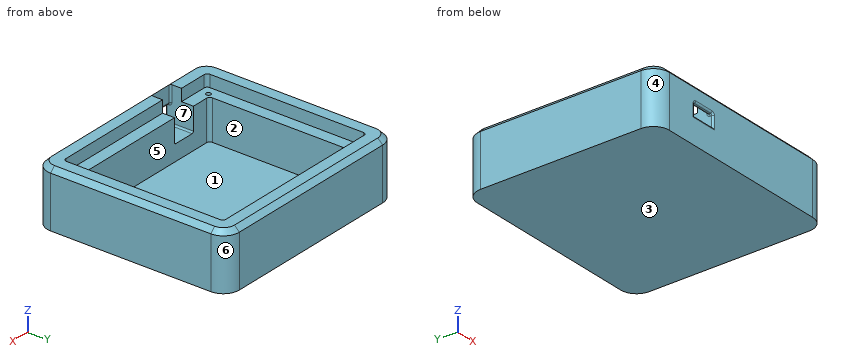
```python
from build123d import *

# Parameters (mm, degrees)
BASE_W              = 134
BASE_H              = 120.5
BASE_W_2            = 114
BASE_H_2            = 100.5
BASE_R              = 1.475
BASE_W_3            = 99
BASE_H_3            = 85.5
BOSS_EXTRUDE1_DEPTH = 3
BOSS_EXTRUDE2_START = 3
BASE_3_W            = 114
BASE_3_H            = 100.5
BASE_3_R            = 1.475
BASE_3_W_2          = 99
BASE_3_H_2          = 85.5
BOSS_EXTRUDE2_DEPTH = 25
BOSS_EXTRUDE3_START = 3
BASE_4_W            = 134
BASE_4_H            = 120.5
BASE_4_W_2          = 114
BASE_4_H_2          = 100.5
BOSS_EXTRUDE3_DEPTH = 32.5
SKETCH2_W           = 15
SKETCH2_H           = 14.5
CUT_EXTRUDE1_DEPTH  = 22.5
SKETCH3_W           = 15
SKETCH3_H           = 8
CUT_EXTRUDE2_DEPTH  = 3
FILLET1_R           = 10
FILLET2_R           = 2
FILLET3_R           = 1
CHAMFER1_SIZE       = 3


with BuildPart() as part:
    # Base → Boss-Extrude1 (new body)
    # profile 1 of 7: a face of its own
    with BuildSketch(Plane.XY):
        Rectangle(BASE_W, BASE_H)
        Rectangle(BASE_W_2, BASE_H_2, mode=Mode.SUBTRACT)
    # profile 2 of 7: a face of its own
    with BuildSketch(Plane.XY):
        Rectangle(BASE_W_2, BASE_H_2)
        with Locations((-51.5, -44.75)):
            Circle(BASE_R, mode=Mode.SUBTRACT)
        with Locations((51.5, -44.75)):
            Circle(BASE_R, mode=Mode.SUBTRACT)
        with Locations((51.5, 44.75)):
            Circle(BASE_R, mode=Mode.SUBTRACT)
        with Locations((-51.5, 44.75)):
            Circle(BASE_R, mode=Mode.SUBTRACT)
        Rectangle(BASE_W_3, BASE_H_3, mode=Mode.SUBTRACT)
    # profile 3 of 7: a face of its own
    with BuildSketch(Plane.XY):
        with Locations((51.5, -44.75)):
            Circle(BASE_R)
    # profile 4 of 7: a face of its own
    with BuildSketch(Plane.XY):
        with Locations((-51.5, 44.75)):
            Circle(BASE_R)
    # profile 5 of 7: a face of its own
    with BuildSketch(Plane.XY):
        with Locations((-51.5, -44.75)):
            Circle(BASE_R)
    # profile 6 of 7: a face of its own
    with BuildSketch(Plane.XY):
        with Locations((51.5, 44.75)):
            Circle(BASE_R)
    # profile 7 of 7: a face of its own
    with BuildSketch(Plane.XY):
        Rectangle(BASE_W_3, BASE_H_3)
    extrude(amount=BOSS_EXTRUDE1_DEPTH)

    # Base<3> → Boss-Extrude2 (add)
    with BuildSketch(Plane.XY.offset(BOSS_EXTRUDE2_START)):
        Rectangle(BASE_3_W, BASE_3_H)
        with Locations((-51.5, -44.75)):
            Circle(BASE_3_R, mode=Mode.SUBTRACT)
        with Locations((51.5, -44.75)):
            Circle(BASE_3_R, mode=Mode.SUBTRACT)
        with Locations((51.5, 44.75)):
            Circle(BASE_3_R, mode=Mode.SUBTRACT)
        with Locations((-51.5, 44.75)):
            Circle(BASE_3_R, mode=Mode.SUBTRACT)
        Rectangle(BASE_3_W_2, BASE_3_H_2, mode=Mode.SUBTRACT)
    extrude(amount=BOSS_EXTRUDE2_DEPTH)

    # Base<4> → Boss-Extrude3 (add)
    with BuildSketch(Plane.XY.offset(BOSS_EXTRUDE3_START)):
        Rectangle(BASE_4_W, BASE_4_H)
        Rectangle(BASE_4_W_2, BASE_4_H_2, mode=Mode.SUBTRACT)
    extrude(amount=BOSS_EXTRUDE3_DEPTH)

    # Sketch2 → Cut-Extrude1 (cut)
    with BuildSketch(Plane.XY.offset(35.5)):
        with Locations((-29.5, -50)):
            Rectangle(SKETCH2_W, SKETCH2_H)
    extrude(amount=-CUT_EXTRUDE1_DEPTH, mode=Mode.SUBTRACT)

    # Sketch3 → Cut-Extrude2 (cut)
    with BuildSketch(Plane.XZ.offset(60.25)):
        with Locations((-29.5, 20.5)):
            Rectangle(SKETCH3_W, SKETCH3_H)
    extrude(amount=-CUT_EXTRUDE2_DEPTH, mode=Mode.SUBTRACT)

    # Fillet1
    fillet1_edges = [part.edges().sort_by_distance(p)[0] for p in [
        (67, 60.25, 17.75),
        (67, -60.25, 17.75),
        (-67, -60.25, 17.75),
        (-67, 60.25, 17.75),
    ]]
    fillet(fillet1_edges, radius=FILLET1_R)

    # Fillet2
    fillet2_edges = [part.edges().sort_by_distance(p)[0] for p in [
        (49.5, -42.75, 15.5),
        (49.5, 42.75, 15.5),
        (-49.5, 42.75, 15.5),
        (-49.5, -42.75, 15.5),
        (57, 50.25, 31.75),
        (-57, -50.25, 31.75),
        (57, -50.25, 31.75),
        (-57, 50.25, 31.75),
    ]]
    fillet(fillet2_edges, radius=FILLET2_R)

    # Fillet3
    fillet3_edges = [part.edges().sort_by_distance(p)[0] for p in [
        (-22, -57.25, 30),
        (-37, -57.25, 30),
        (-37, -60.25, 20.5),
        (-22, -60.25, 20.5),
        (-29.5, -57.25, 24.5),
        (-37, -58.75, 24.5),
        (-29.5, -60.25, 24.5),
        (-22, -58.75, 24.5),
        (-37, -50, 13),
        (-22, -50, 13),
        (-29.5, -60.25, 16.5),
    ]]
    fillet(fillet3_edges, radius=FILLET3_R)

    # Chamfer1
    chamfer1_edges = [part.edges().sort_by_distance(p)[0] for p in [
        (0, 60.25, 35.5),
        (67, 0, 35.5),
        (0, -60.25, 35.5),
        (-67, 0, 35.5),
        (64.071067812, -57.321067812, 35.5),
        (-64.071067812, -57.321067812, 35.5),
        (-64.071067812, 57.321067812, 35.5),
        (64.071067812, 57.321067812, 35.5),
    ]]
    chamfer(chamfer1_edges, length=CHAMFER1_SIZE - 0.0001)  # a hair under: the kernel refuses the full size


solid = part.part
```
Geometry check sheet. Reference: the model listing, model coordinates, mm. Face numbers are marked on the shaded views. A direction names the side the tool comes from. Give positions to 0.01 mm unless a question says otherwise; leave off trailing zeros. Loops run counter-clockwise (first coordinate to the right, second up) from the corner with the lowest first, then second, coordinate; pieces in that order, holes last. Notation, with made-up numbers: M 89.5,55 L 122.5,55 A31 ccw 122.5,87 Z; hole C 8.5,54 d3. An arc over 180 degrees is marked long. Write item = value, one per line.
(1) Sectioned sample at B-B, the plane z = 20.5. Record the cut outline in (x, y) (3 decimals), plus the area to 3 significant figures.
Answer below:
outline = M -67,-50.25 A10 ccw -57,-60.25 L -38,-60.25 A1 ccw -37,-59.25 L -37,-42.75 L -47.5,-42.75 A2 cw -49.5,-40.75 L -49.5,40.75 A2 cw -47.5,42.75 L 47.5,42.75 A2 cw 49.5,40.75 L 49.5,-40.75 A2 cw 47.5,-42.75 L -22,-42.75 L -22,-59.25 A1 ccw -21,-60.25 L 57,-60.25 A10 ccw 67,-50.25 L 67,50.25 A10 ccw 57,60.25 L -57,60.25 A10 ccw -67,50.25 Z; hole C -51.5,-44.75 d2.95; hole C -51.5,44.75 d2.95; hole C 51.5,-44.75 d2.95; hole C 51.5,44.75 d2.95
area = 7,310 mm2
(2) Release check for a two-part mould opening along X. For the marked faces 1, 2, 3 and 4 record: released by +X, released by -X, zero draft, split by the parting line, or undercut.
Answer below:
face_1 = undercut
face_2 = undercut
face_3 = zero draft
face_4 = released by -X
(3) Sectioned sample at D-D, the plane z = 11. Record the cut outline in (x, y) (3 decimals).
Answer below:
outline = M -67,-50.25 A10 ccw -57,-60.25 L 57,-60.25 A10 ccw 67,-50.25 L 67,50.25 A10 ccw 57,60.25 L -57,60.25 A10 ccw -67,50.25 Z; hole C -51.5,-44.75 d2.95; hole C -51.5,44.75 d2.95; hole M -49.5,-40.75 A2 ccw -47.5,-42.75 L 47.5,-42.75 A2 ccw 49.5,-40.75 L 49.5,40.75 A2 ccw 47.5,42.75 L -47.5,42.75 A2 ccw -49.5,40.75 Z; hole C 51.5,-44.75 d2.95; hole C 51.5,44.75 d2.95
(4) Gauge pin test, flat end, axial feed: pin 1 Ø3 at (x, y) = (51.5, -44) entering from +Z. Record the tip position at first contact, or that the pin passes through.
Answer below:
pin_1 = 28
(5) Sectioned sample at C-C, the plane y = -44.75. Record the cut outline in (x, z) (3 decimals), plus the area to 3 significant figures.
Answer below:
outline = M -67,0 L 67,0 L 67,32.5 L 64,35.5 L 57,35.5 L 57,28 L 52.975,28 L 52.975,3 L 50.025,3 L 50.025,28 L -22,28 L -22,14 A1 cw -23,13 L -36,13 A1 cw -37,14 L -37,28 L -50.025,28 L -50.025,3 L -52.975,3 L -52.975,28 L -57,28 L -57,35.5 L -64,35.5 L -67,32.5 Z
area = 3,520 mm2
(6) Material ranges on line 1 (Y direction, x = 51.5, z = 21.5) (3 decimals); line 2 (Y direction, x = 11.5, z = 11.5); line 3 (X direction, y = -28.5, z = 9.5), recorded low to high. Write a range as [from, to].
Answer below:
line_1 = [-60.25, -46.225], [-43.275, 43.275], [46.225, 60.25]
line_2 = [-60.25, -42.75], [42.75, 60.25]
line_3 = [-67, -49.5], [49.5, 67]
(7) Tool access check on the marked faces 5, 6 and 7. Record the directions out of +Z, -Z, +X, -X, +Y, -Y that give a thin tool (end or side, any length) a straight path to the whole face; none if there is none.
Answer below:
face_5 = +Z
face_6 = +Z, -Z, +X, +Y
face_7 = none
